Input: part model. Units: mm. Frame: model coordinates. A direction names the side the tool comes from. Give positions to 0.01 mm unless a question says otherwise; leave off trailing zeros. Loops run counter-clockwise (first coordinate to the right, second up) from the corner with the lowest first, then second, coordinate; pieces in that order, holes last. Notation, with made-up numbers: (-2.5, 36) -> (17.5, 36) arc R27 ccw to (17.5, 61) -> close; hole circle Ø1 at (8, 15.25). An arc over 180 degrees is marked (long way). Answer as a JSON object with one key per item and string values. Group by question number.
```python
from build123d import *

# Parameters (mm, degrees)
CUT_EXTRUDE_1_DEPTH = 3
FILLET_1_R          = 0.3
CHAMFER_1_SIZE      = 1


with BuildPart() as part:
    # Эскиз1 → Повернуть1 (revolve)
    with BuildSketch(Plane.XY, mode=Mode.PRIVATE) as revolve_1_sk:
        Polygon((0, 0), (0, 5.9), (0.5, 5.9), (4, 3), (20, 3), (20, 0), align=None)
    revolve(revolve_1_sk.sketch.rotate(Axis((0, 0, 0), (1, 0, 0)), 90), axis=Axis((0, 0, 0), (1, 0, 0)))  # turned: the seam where the file's is

    # Эскиз2 → Вырез-Вытянуть1 (cut)
    with BuildSketch(Plane.ZY):
        Polygon((1.154700538, 2), (-1.154700538, 2), (-2.309401077, 0), (-1.154700538, -2), (1.154700538, -2), (2.309401077, 0), align=None)
    extrude(amount=-CUT_EXTRUDE_1_DEPTH, mode=Mode.SUBTRACT)

    # Скругление1
    fillet_1_edges = [part.edges().sort_by_distance(p)[0] for p in [
        (0, 0, -5.9),
    ]]
    fillet(fillet_1_edges, radius=FILLET_1_R)

    # Фаска1
    chamfer_1_edges = [part.edges().sort_by_distance(p)[0] for p in [
        (20, 0, -3),
    ]]
    chamfer(chamfer_1_edges, length=CHAMFER_1_SIZE)


solid = part.part
```
Q1. Pull-direction query (Y, two-part tool) for faces 1 (the face through (0, 2.4, 0.1)), 2 (the face through (11.6, -0.9, 2.86)), 3 (the face through (3, 0, 0)); classes: +Y half, -Y half, draft (parallel to the pull), parting line (faces both ways), or undercut.
Q2. Ray query, probe 1 along X at (y, z) = (4.5, -2); probe 2 along Z at (x, y) = (14.75, 2.75); probe 3 along X at (y, z) = (-2, -3.25). Return the intervals inside material, ascending.
Q3. Section B-B on x = 5.5. Return the cut outline in (y, z).
Q4. Set-up query: faces 4 (the face through (1.48, 0.99, 1.74)), 5 (the face through (3.83, -0.943, 2.996)). Return all of +Z, -Z, +X, -X, +Y, -Y with unobstructed straight access to the full face (end or side cutting, diameter ignored); none if empty.
Q5. Section A-A on z = 0. Return the cut outline in (x, y).
Q6. Pin query (flat end, axial travel): pin 1 Ø4 at (x, z) = (7.5, 4) entering from +Y; pin 2 Ø2 at (x, y) = (11, 1.5) entering from -Z; pin 3 Ø5 at (x, z) = (11, -1) entering from +Y. Return the tip coordinate at first contact, or that it passes through.
Numbers:
{
 "1": {"face 1": "draft", "face 2": "parting line", "face 3": "undercut"},
 "2": {"probe 1": "x = 0 to 1.68", "probe 2": "z = -1.2 to 1.2", "probe 3": "x = 0 to 3.02"},
 "3": {"outline": "circle Ø6 at (0, 0)"},
 "4": {"face 4": "-X", "face 5": "+X"},
 "5": {"outline": "(0, -5.6) arc R0.3 ccw to (0.3, -5.9) -> (0.5, -5.9) -> (4, -3) -> (19, -3) -> (20, -2) -> (20, 2) -> (19, 3) -> (4, 3) -> (0.5, 5.9) -> (0.3, 5.9) arc R0.3 ccw to (0, 5.6) -> (0, 2) -> (3, 2) -> (3, -2) -> (0, -2) -> close"},
 "6": {"pin 1": "stops at y = 2.24", "pin 2": "stops at z = -2.96", "pin 3": "stops at y = 3"}
}
